The drawing under review shows one solid part. Ordinate dimensions are in mm from its lowest x, y, z. Coordinates: 2 decimals unless noted, no trailing zeros. Write each loop counter-clockwise with the first axis right and the second up, starting at its lowest first coordinate (ties: lowest second). Pieces come first, ordered by that corner, then holes.
Q1. Take a section at B-B (y = 1.5). Give the boundary of the cut face in (x, z), and give its area (3 significant figures).
Q2. Take a section at A-A (z = 323.5). Give the boundary of the cut face in (x, y), and give its area (3 significant figures).
Q3. Insertion check: pin 1 (1.9 mm diameter, centred on y = 2.5, z = 220, fed in from -X). The pin has a flat end and moves straight along its axis. Give the tip position at first contact, or say it passes through.
Q4. For probe 1 along X at (y, z) = (5.25, 57); probe 2 along X at (y, z) = (1.5, 48.5), list the stretches that pass through material, from the lowest coordinate up.
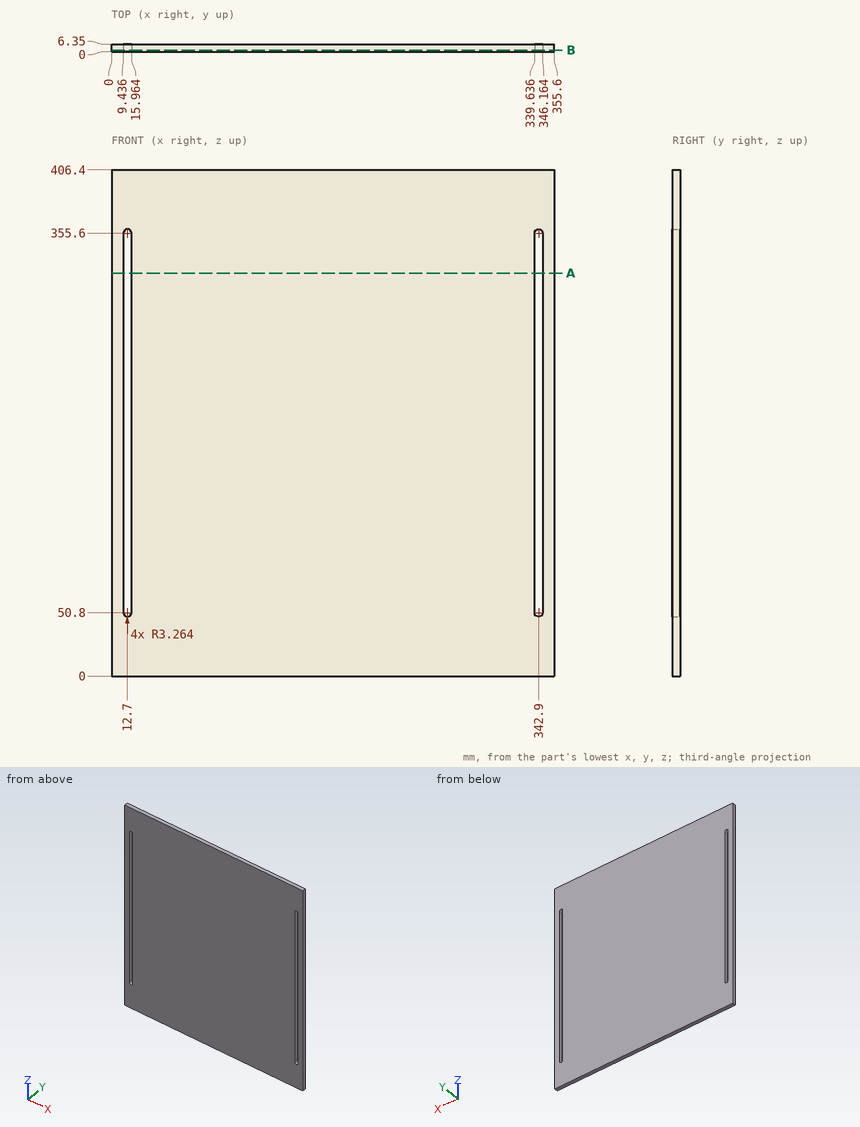
Response:
1. outline: (0, 0) - (355.6, 0) - (355.6, 406.4) - (0, 406.4) - close; hole (9.44, 50.8) arc R3.26 ccw to (15.96, 50.8) - (15.96, 355.6) arc R3.26 ccw to (9.44, 355.6) - close; hole (339.64, 50.8) arc R3.26 ccw to (346.16, 50.8) - (346.16, 355.6) arc R3.26 ccw to (339.64, 355.6) - close
1. area: 140,000 mm2
2. outline: (0, 0) - (9.44, 0) - (9.44, 6.35) - (0, 6.35) - close; (15.96, 0) - (339.64, 0) - (339.64, 6.35) - (15.96, 6.35) - close; (346.16, 0) - (355.6, 0) - (355.6, 6.35) - (346.16, 6.35) - close
2. area: 2,180 mm2
3. pin 1: stops at x = 0
4. probe 1: x = 0 to 9.44, 15.96 to 339.64, 346.16 to 355.6
4. probe 2: x = 0 to 10.38, 15.02 to 340.58, 345.22 to 355.6
